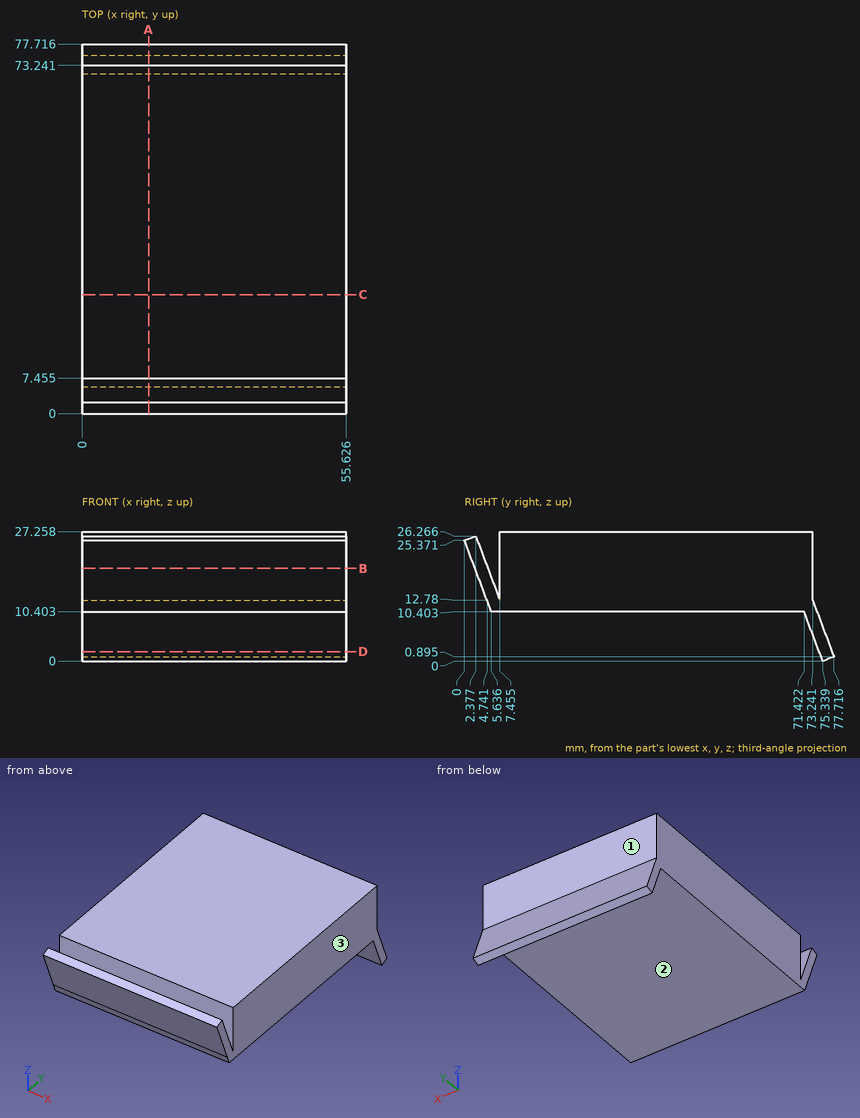
The drawing under review shows one solid part. Ordinate dimensions are in mm from its lowest x, y, z. A direction names the side the tool comes from. Coordinates: 2 decimals unless noted, no trailing zeros. Write each loop counter-clockwise with the first axis right and the second up, starting at its lowest first coordinate (ties: lowest second). Pieces come first, ordered by that corner, then holes.
1) Add section C-C (y = 25). Write out the cut boundary in (x, z).
2) Add section B-B (z = 19.5). Write out the cut boundary in (x, y) (1 decimal), plus the area to 3 significant figures.
3) Add section A-A (x = 14). Write out the cut boundary in (y, z) (1 decimal).
4) Machinability: for the marked faces 1, 2 and 3, which of the approach directions +Z, -Z, +X, -X, +Y, -Y give a long, thin tool a straight path to every point of the face, cutting with its end or side? Answer none if there is none.
5) To check wall thickness, follow L1, parallel to Z at x = 32, y = 68; L2, parallel to Y at x = 10, z = 17 (1 decimal); L3, parallel to Y at x = 24, z = 14 (1 decimal). State the ranges of each line that lie inside material, in increasing order.
6) Insertion check: pin 1 (6 mm diameter, centred on x = 44, z = 13, fed in from -Y); pin 2 (2 mm diameter, centred on y = 38, z = 11, fed in from -X); pin 3 (4 mm diameter, centred on x = 34, z = 8, fed in from -Y); pin 4 (11.5 mm diameter, centred on x = 22, z = 18, fed in from -Y). Each pin has a flat end and moves straight along its axis. Give the tip position at first contact, or say it passes through.
7) Add section D-D (z = 2). Write out the cut boundary in (x, y).
Check result:
1. outline: (0, 10.4) - (55.63, 10.4) - (55.63, 27.26) - (0, 27.26) - close
2. outline: (0, 2.2) - (55.6, 2.2) - (55.6, 4.9) - (0, 4.9) - close; (0, 7.5) - (55.6, 7.5) - (55.6, 73.2) - (0, 73.2) - close
2. area: 3,810 mm2
3. outline: (0, 25.4) - (4.7, 12.8) - (5.6, 10.4) - (71.4, 10.4) - (75.3, 0) - (77.7, 0.9) - (73.2, 12.8) - (73.2, 27.3) - (7.5, 27.3) - (7.5, 12.8) - (2.4, 26.3) - close
4. face 1: +Z, +X, -X, +Y
4. face 2: -Z, +X, -X, -Y
4. face 3: +Z, -Z, +X, +Y, -Y
5. L1: z = 10.4 to 27.26
5. L2: y = 3.2 to 5.9, 7.5 to 73.2
5. L3: y = 4.3 to 7, 7.5 to 73.2
6. pin 1: stops at y = 3.53
6. pin 2: stops at x = 0
6. pin 3: stops at y = 71.57
6. pin 4: stops at y = 0.61
7. outline: (0, 74.59) - (55.63, 74.59) - (55.63, 77.3) - (0, 77.3) - close
